Study the drawing (mm; zero at the part's minimum x, y, z) and answer. A direction names the side the tool comes from. Give positions to 0.01 mm unless a question says otherwise; leave off trailing zeros. Write each loop counter-clockwise with the first axis right and the second up, starting at its lowest first coordinate (ties: lowest second). Pieces come first, ordered by that corner, then holes. Notation, with made-up numbers: (-4.75, -37) - (20.25, -37) arc R7 cw to (20.25, -26) - close; hole circle Ø10 at (-31.5, -11). An arc over 180 degrees is marked (long way). Write each question's results on one line, items separated by ' | '. Start each with the question number.
Q1. For a pull along Y with two mould halves and no side action, classify the marked faces 3, 4 and 5 as pulls with the +Y half, pulls with the -Y half, needs draft (parallel to the pull), parting line crosses it, or undercut.
Q2. Section C-C (z = 19.5) is taken. Determine the outline of the cut face in (x, y).
Q3. Section A-A (x = 36) is taken. Determine the outline of the cut face in (y, z) (1 decimal).
Q4. Find the intervals of material crossed by probe 1 along Z at (x, y) = (27.5, 27) (1 decimal); probe 2 along Y at (x, z) = (30, 31); probe 3 along X at (y, z) = (34, 17), in increasing order.
Q5. Flat-ended cylindrical pins translate along their axes: pin 1 Ø4 at (x, y) = (34, 15.5) entering from -Z; pin 2 Ø14 at (y, z) = (26, 28) entering from +X. Find the tip coordinate at first contact, or state that the pin passes through.
Q6. For the marked faces 1 and 2, determine the directions among +Z, -Z, +X, -X, +Y, -Y from which every point of the face is accessible in a straight line to the end or side of a thin tool.
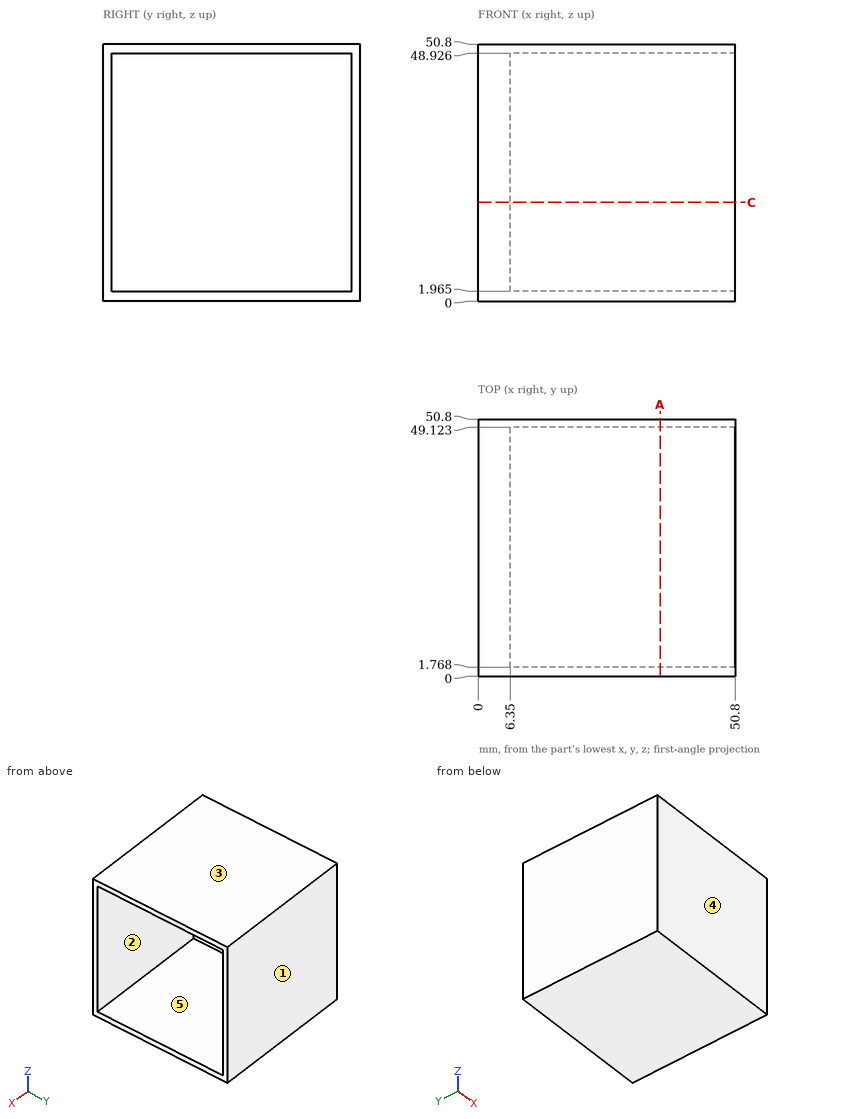
Answers below:
1) face 3: needs draft | face 4: pulls with the -Y half | face 5: undercut
2) outline: (0, 0) - (50.8, 0) - (50.8, 1.77) - (6.35, 1.77) - (6.35, 49.12) - (50.8, 49.12) - (50.8, 50.8) - (0, 50.8) - close
3) outline: (0, 0) - (50.8, 0) - (50.8, 50.8) - (0, 50.8) - close; hole (1.8, 2) - (49.1, 2) - (49.1, 48.9) - (1.8, 48.9) - close
4) probe 1: z = 0 to 2, 48.9 to 50.8 | probe 2: y = 0 to 1.77, 49.12 to 50.8 | probe 3: x = 0 to 6.35
5) pin 1: stops at z = 0 | pin 2: stops at x = 6.35
6) face 1: +Z, -Z, +X, -X, +Y | face 2: +X
